Read the model definition and answer for the solid it produces. Units are mm, in the model's axes. A direction names the side the tool comes from. Coordinates: 2 decimals unless noted, no trailing zeros. Write each loop counter-clockwise with the first axis right and the second up, starting at its lowest first coordinate (ties: lowest second). Pieces come first, ordered by that corner, then holes.
(1) Given pin 1 (2 mm diameter, centred on y = 1, z = 8, fed in from +X); pin 2 (2 mm diameter, centred on x = -9, y = -0.5, fed in from +Z); pin 3 (0.6 mm diameter, centred on y = 1, z = -1.5, fed in from -X), each flat-ended and moving along its own axis, determine where each tip first touches the part or whether it passes through.
(2) The part is cut by section C-C, the plane y = -3.5. Determine the outline of the cut face in (x, z).
(3) Determine the mould class of faces 5 (the flat face through (10.5, -1, 1)), 6 (the flat face through (-12.5, 0, 0)), 7 (the flat face through (-1, -12.5, 1)) for opening direction Y: pulls with the +Y half, pulls with the -Y half, needs draft (parallel to the pull), parting line crosses it, or undercut.
(4) Which of the six approach directions +Z, -Z, +X, -X, +Y, -Y give full straight-line access (tool end or side, diameter ignored) to faces 1 (the flat face through (12.5, 0, 0)), 2 (the cylindrical face through (-0.594, -3.94, -40.026)), 3 (the flat face through (-9.8, 0.3, 17.5)), 4 (the flat face through (5.75, 1, 10))?
(5) The part is cut by section B-B, the plane x = 0. Determine the outline of the cut face in (y, z), and give its area (3 significant figures).
(6) The part is cut by section D-D, the plane z = -1. Determine the outline of the cut face in (x, y).
(7) The part is cut by section A-A, the plane z = -35.5. Determine the outline of the cut face in (x, y).
(8) Straight lines are drawn through the part: line 1 along Z through (x, y) = (0, -8.25); line 2 along Z through (x, y) = (0, -3.8); line 3 along X through (y, z) = (-7.5, 35.5). For each, find the intervals that lie inside material, in ascending order.
```python
from build123d import *

# Parameters (mm, degrees)
BOSS_EXTRUDE1_DEPTH                             = 2
BOSS_EXTRUDE2_DEPTH                             = 2.5
SKETCH3_W                                       = 75
SKETCH3_H                                       = 90
BOSS_EXTRUDE3_DEPTH                             = 10
CBORE_FOR_8_PAN_HEAD_MACHINE_SCREW1_D           = 4.9784
CBORE_FOR_8_PAN_HEAD_MACHINE_SCREW1_CBORE_D     = 9.12876
CBORE_FOR_8_PAN_HEAD_MACHINE_SCREW1_CBORE_DEPTH = 2.921


with BuildPart() as part:
    # Sketch1 → Boss-Extrude1 (new body)
    with BuildSketch(Plane(origin=(0, 0, 0), x_dir=(1, 0, 0), z_dir=(0, 1, 0))):
        Polygon((12.5, 17.5), (-12.5, 17.5), (-12.5, -17.5), (-5.75, -17.5), (-5.75, -2.5), (-4.25, -2.5), (-4.25, 7.5), (4.25, 7.5), (4.25, -2.5), (5.75, -2.5), (5.75, -17.5), (12.5, -17.5), align=None)
    extrude(amount=BOSS_EXTRUDE1_DEPTH)

    # Sketch2 → Boss-Extrude2 (add)
    with BuildSketch(Plane.XZ):
        Polygon((-12.5, 17.5), (-12.5, -17.5), (12.5, -17.5), (12.5, 17.5), (10.5, 17.5), (10.5, -15.5), (-10.5, -15.5), (-10.5, 17.5), align=None)
    extrude(amount=BOSS_EXTRUDE2_DEPTH)

    # Sketch3 → Boss-Extrude3 (add)
    with BuildSketch(Plane.XZ.offset(2.5)):
        Rectangle(SKETCH3_W, SKETCH3_H)
    extrude(amount=BOSS_EXTRUDE3_DEPTH)

    # CBORE for #8 Pan Head Machine Screw1 (through all)
    with Locations(Plane(origin=(0, -2.5, 0), x_dir=(1, 0, 0), z_dir=(0, 1, 0))):
        with Locations((0, 35.5), (0, -35.5)):
            CounterBoreHole(CBORE_FOR_8_PAN_HEAD_MACHINE_SCREW1_D / 2, CBORE_FOR_8_PAN_HEAD_MACHINE_SCREW1_CBORE_D / 2, CBORE_FOR_8_PAN_HEAD_MACHINE_SCREW1_CBORE_DEPTH)


solid = part.part
```
Computed:
1. pin 1: stops at x = 12.5
1. pin 2: stops at z = 17.5
1. pin 3: stops at x = -12.5
2. outline: (-37.5, -45) - (37.5, -45) - (37.5, 45) - (-37.5, 45) - close; hole circle Ø9.13 at (0, -35.5); hole circle Ø9.13 at (0, 35.5)
3. face 5: undercut
3. face 6: needs draft
3. face 7: pulls with the -Y half
4. face 1: +Z, -Z, +X, +Y
4. face 2: +Y
4. face 3: +Z, +X, -X, +Y
4. face 4: +Z, +Y
5. outline: (-12.5, -45) - (-2.5, -45) - (-2.5, -40.06) - (-5.42, -40.06) - (-5.42, -37.99) - (-12.5, -37.99) - close; (-12.5, -33.01) - (-5.42, -33.01) - (-5.42, -30.94) - (-2.5, -30.94) - (-2.5, -17.5) - (2, -17.5) - (2, -7.5) - (0, -7.5) - (0, -15.5) - (-2.5, -15.5) - (-2.5, 30.94) - (-5.42, 30.94) - (-5.42, 33.01) - (-12.5, 33.01) - close; (-12.5, 37.99) - (-5.42, 37.99) - (-5.42, 40.06) - (-2.5, 40.06) - (-2.5, 45) - (-12.5, 45) - close
5. area: 801 mm2
6. outline: (-37.5, -12.5) - (37.5, -12.5) - (37.5, -2.5) - (12.5, -2.5) - (12.5, 2) - (4.25, 2) - (4.25, 0) - (10.5, 0) - (10.5, -2.5) - (-10.5, -2.5) - (-10.5, 0) - (-4.25, 0) - (-4.25, 2) - (-12.5, 2) - (-12.5, -2.5) - (-37.5, -2.5) - close
7. outline: (-37.5, -12.5) - (-2.49, -12.5) - (-2.49, -5.42) - (-4.56, -5.42) - (-4.56, -2.5) - (-37.5, -2.5) - close; (2.49, -12.5) - (37.5, -12.5) - (37.5, -2.5) - (4.56, -2.5) - (4.56, -5.42) - (2.49, -5.42) - close
8. line 1: z = -45 to -37.99, -33.01 to 33.01, 37.99 to 45
8. line 2: z = -45 to -40.06, -30.94 to 30.94, 40.06 to 45
8. line 3: x = -37.5 to -2.49, 2.49 to 37.5
